Check sheet for the modelled part. Datum: model origin and axes. Units: mm. A direction names the side the tool comes from. Round coordinates to 2 decimals unless told otherwise and drop trailing zeros. Loops run counter-clockwise (first coordinate to the right, second up) from the corner with the lowest first, then second, coordinate; pieces in that order, holes last. Notation, with made-up numbers: (17.5, 24) -> (30.5, 24) arc R15 cw to (30.5, 46) -> close; hole circle Ø10 at (21.25, 10.25). An arc over 180 degrees is marked (long way). One line per question, with ' | ' between items.
```python
from build123d import *

# Parameters (mm, degrees)
SKETCH1_R               = 6
BOSS_EXTRUDE1_DEPTH     = 25.8
CHAMFER1_SIZE           = 1.6
SKETCH2_W               = 3.15
SKETCH2_H               = 10.8
CUT_EXTRUDE1_DEPTH      = 7
CUT_EXTRUDE1_DEPTH_BACK = 7
SKETCH3_R               = 2.25
CUT_EXTRUDE2_DEPTH      = 4.15
CUT_EXTRUDE2_DEPTH_BACK = 9.85
SKETCH4_R               = 2.25
CUT_EXTRUDE3_DEPTH      = 7
CUT_EXTRUDE3_DEPTH_BACK = 7


with BuildPart() as part:
    # Sketch1 → Boss-Extrude1 (new body)
    with BuildSketch(Plane(origin=(0, 0, 0), x_dir=(1, 0, 0), z_dir=(0, 1, 0))):
        Circle(SKETCH1_R)
    extrude(amount=-BOSS_EXTRUDE1_DEPTH)

    # Chamfer1
    chamfer1_edges = [part.edges().sort_by_distance(p)[0] for p in [
        (-6, 0, 0),
    ]]
    chamfer(chamfer1_edges, length=CHAMFER1_SIZE)

    # Sketch2 → Cut-Extrude1 (cut, two sides)
    with BuildSketch(Plane(origin=(0, 0, 0), x_dir=(0, 0, -1), z_dir=(1, 0, 0))) as cut_extrude1_sk:
        with Locations((4.425, -20.4)):
            Rectangle(SKETCH2_W, SKETCH2_H)
        with Locations((-4.425, -20.4)):
            Rectangle(SKETCH2_W, SKETCH2_H)
    extrude(amount=CUT_EXTRUDE1_DEPTH, mode=Mode.SUBTRACT)
    extrude(cut_extrude1_sk.sketch, amount=-CUT_EXTRUDE1_DEPTH_BACK, mode=Mode.SUBTRACT)

    # Sketch3 → Cut-Extrude2 (cut, two sides)
    with BuildSketch(Plane.XY.offset(2.85)) as cut_extrude2_sk:
        with Locations((0, -20.4)):
            Circle(SKETCH3_R)
    extrude(amount=CUT_EXTRUDE2_DEPTH, mode=Mode.SUBTRACT)
    extrude(cut_extrude2_sk.sketch, amount=-CUT_EXTRUDE2_DEPTH_BACK, mode=Mode.SUBTRACT)

    # Sketch4 → Cut-Extrude3 (cut, two sides)
    with BuildSketch(Plane(origin=(0, 0, 0), x_dir=(0, 0, -1), z_dir=(1, 0, 0))) as cut_extrude3_sk:
        with Locations((0, -7.4)):
            Circle(SKETCH4_R)
    extrude(amount=CUT_EXTRUDE3_DEPTH, mode=Mode.SUBTRACT)
    extrude(cut_extrude3_sk.sketch, amount=-CUT_EXTRUDE3_DEPTH_BACK, mode=Mode.SUBTRACT)


solid = part.part
```
(1) Set-up check for faces 5 (the face through (-2.4, -20.5, 2.85)), 6 (the face through (0, -15, -4)), 7 (the face through (5.54, -10.84, 2.3)): record each of +Z, -Z, +X, -X, +Y, -Y from which the full face is reachable in a straight line by a thin tool's end or side.
Answer:
face 5: +Z, +X, -X, -Y | face 6: -Z, +X, -X, -Y | face 7: +Y, -Y
(2) Scan lines: probe 1 along Y at (x, z) = (-1.25, 0); probe 2 along Y at (x, z) = (0, 0.95); probe 3 along Y at (x, z) = (1.25, 3). Record each from-to range of solid material in increasing order.
Answer:
probe 1: y = -25.8 to -22.27, -18.53 to -9.65, -5.15 to 0 | probe 2: y = -25.8 to -22.65, -18.15 to -9.44, -5.36 to 0 | probe 3: y = -15 to 0
(3) Sectioned sample at B-B, the plane z = 0.5. Count the separate pieces of the cut face and the enclosed holes in it, and give its area (3 significant figures).
Answer:
separate pieces: 2 | enclosed holes: 1 | area: 238 mm2
(4) Sectioned sample at D-D, the plane y = -23. Record the cut outline in (x, z), and give its area (3 significant figures).
Answer:
outline: (-5.28, -2.85) -> (5.28, -2.85) arc R6 ccw to (5.28, 2.85) -> (-5.28, 2.85) arc R6 ccw to start | area: 65.7 mm2
(5) Mould release check, pull along Y, two halves, no side actions. Record for faces 1 (the face through (0, -25.8, 0)), 2 (the face through (2.4, -20.5, -2.85)), 3 (the face through (-0.29, -18.17, 0.04)), 4 (the face through (0, 0, 0)): +Y half, -Y half, draft (parallel to the pull), parting line (faces both ways), or undercut.
Answer:
face 1: -Y half | face 2: draft | face 3: undercut | face 4: +Y half
(6) Sectioned sample at C-C, the plane y = -3.25. Record the cut outline in (x, z).
Answer:
outline: circle Ø12 at (0, 0)
(7) Go/stop test with flat-tipped pins: pin 1 (0.9 mm diameter, centred on x = 0, z = -4, fed in from -Y); pin 2 (1 mm diameter, centred on x = -3.5, y = -21, fed in from +Z); pin 3 (5.5 mm diameter, centred on x = -2.5, y = -22, fed in from -Z). Record where each tip stops, or that it passes through.
Answer:
pin 1: stops at y = -15 | pin 2: stops at z = 2.85 | pin 3: stops at z = -2.85
(8) Sectioned sample at A-A, the plane y = -20.4. Record the cut outline in (x, z).
Answer:
outline: (-5.28, -2.85) -> (-2.25, -2.85) -> (-2.25, 2.85) -> (-5.28, 2.85) arc R6 ccw to start; (2.25, -2.85) -> (5.28, -2.85) arc R6 ccw to (5.28, 2.85) -> (2.25, 2.85) -> close
